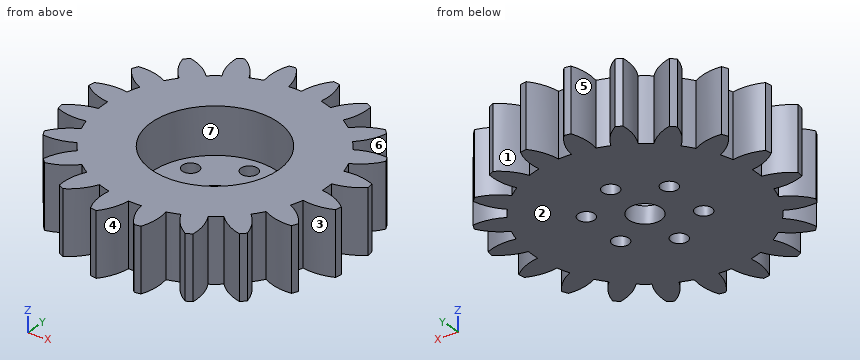
```python
from build123d import *

# Parameters (mm, degrees)
SKETCH1_R           = 3.25
BOSS_EXTRUDE1_DEPTH = 12.7
CUT_EXTRUDE1_REACH  = 43.167
SKETCH2_R           = 1.651
SKETCH3_R           = 12.7
CUT_EXTRUDE2_DEPTH  = 9.271


with BuildPart() as part:
    # Sketch1 → Boss-Extrude1 (new body)
    with BuildSketch(Plane.XY):
        with BuildLine():
            ThreePointArc((-27.689807384, 3.730705969), (-25.124393342, 2.086949602), (-22.186968024, 1.277742146))
            ThreePointArc((-22.186968024, 1.277742146), (-22.22373, 0), (-22.186968024, -1.277742146))
            ThreePointArc((-22.186968024, -1.277742146), (-25.124393342, -2.086949602), (-27.689807384, -3.730705969))
            ThreePointArc((-27.689807384, -3.730705969), (-27.596012236, -4.370778953), (-27.487423293, -5.00850883))
            ThreePointArc((-27.487423293, -5.00850883), (-24.539620899, -5.779057498), (-21.495904554, -5.640945179))
            ThreePointArc((-21.495904554, -5.640945179), (-21.136023233, -6.867510248), (-20.706216479, -8.071355168))
            ThreePointArc((-20.706216479, -8.071355168), (-23.249815112, -9.748671534), (-25.181720202, -12.104733275))
            ThreePointArc((-25.181720202, -12.104733275), (-24.894722286, -12.684494563), (-24.594378694, -13.257455889))
            ThreePointArc((-24.594378694, -13.257455889), (-21.552739385, -13.079370185), (-18.700672175, -12.007457487))
            ThreePointArc((-18.700672175, -12.007457487), (-17.979375248, -13.062780745), (-17.198596196, -14.074887709))
            ThreePointArc((-17.198596196, -14.074887709), (-19.099382988, -16.456125574), (-20.208670796, -19.293864949))
            ThreePointArc((-20.208670796, -19.293864949), (-19.756563466, -19.756563466), (-19.293864949, -20.208670796))
            ThreePointArc((-19.293864949, -20.208670796), (-16.456125574, -19.099382988), (-14.074887709, -17.198596196))
            ThreePointArc((-14.074887709, -17.198596196), (-13.062780745, -17.979375248), (-12.007457487, -18.700672175))
            ThreePointArc((-12.007457487, -18.700672175), (-13.079370185, -21.552739385), (-13.257455889, -24.594378694))
            ThreePointArc((-13.257455889, -24.594378694), (-12.684494563, -24.894722286), (-12.104733275, -25.181720202))
            ThreePointArc((-12.104733275, -25.181720202), (-9.748671534, -23.249815112), (-8.071355168, -20.706216479))
            ThreePointArc((-8.071355168, -20.706216479), (-6.867510248, -21.136023233), (-5.640945179, -21.495904554))
            ThreePointArc((-5.640945179, -21.495904554), (-5.779057498, -24.539620899), (-5.00850883, -27.487423293))
            ThreePointArc((-5.00850883, -27.487423293), (-4.370778953, -27.596012236), (-3.730705969, -27.689807384))
            ThreePointArc((-3.730705969, -27.689807384), (-2.086949602, -25.124393342), (-1.277742146, -22.186968024))
            ThreePointArc((-1.277742146, -22.186968024), (0, -22.22373), (1.277742146, -22.186968024))
            ThreePointArc((1.277742146, -22.186968024), (2.086949602, -25.124393342), (3.730705969, -27.689807384))
            ThreePointArc((3.730705969, -27.689807384), (4.370778953, -27.596012236), (5.00850883, -27.487423293))
            ThreePointArc((5.00850883, -27.487423293), (5.779057498, -24.539620899), (5.640945179, -21.495904554))
            ThreePointArc((5.640945179, -21.495904554), (6.867510248, -21.136023233), (8.071355168, -20.706216479))
            ThreePointArc((8.071355168, -20.706216479), (9.748671534, -23.249815112), (12.104733275, -25.181720202))
            ThreePointArc((12.104733275, -25.181720202), (12.684494563, -24.894722286), (13.257455889, -24.594378694))
            ThreePointArc((13.257455889, -24.594378694), (13.079370185, -21.552739385), (12.007457487, -18.700672175))
            ThreePointArc((12.007457487, -18.700672175), (13.062780745, -17.979375248), (14.074887709, -17.198596196))
            ThreePointArc((14.074887709, -17.198596196), (16.456125574, -19.099382988), (19.293864949, -20.208670796))
            ThreePointArc((19.293864949, -20.208670796), (19.756563466, -19.756563466), (20.208670796, -19.293864949))
            ThreePointArc((20.208670796, -19.293864949), (19.099382988, -16.456125574), (17.198596196, -14.074887709))
            ThreePointArc((17.198596196, -14.074887709), (17.979375248, -13.062780745), (18.700672175, -12.007457487))
            ThreePointArc((18.700672175, -12.007457487), (21.552739385, -13.079370185), (24.594378694, -13.257455889))
            ThreePointArc((24.594378694, -13.257455889), (24.894722286, -12.684494563), (25.181720202, -12.104733275))
            ThreePointArc((25.181720202, -12.104733275), (23.249815112, -9.748671534), (20.706216479, -8.071355168))
            ThreePointArc((20.706216479, -8.071355168), (21.136023233, -6.867510248), (21.495904554, -5.640945179))
            ThreePointArc((21.495904554, -5.640945179), (24.539620899, -5.779057498), (27.487423293, -5.00850883))
            ThreePointArc((27.487423293, -5.00850883), (27.596012236, -4.370778953), (27.689807384, -3.730705969))
            ThreePointArc((27.689807384, -3.730705969), (25.124393342, -2.086949602), (22.186968024, -1.277742146))
            ThreePointArc((22.186968024, -1.277742146), (22.22373, 0), (22.186968024, 1.277742146))
            ThreePointArc((22.186968024, 1.277742146), (25.124393342, 2.086949602), (27.689807384, 3.730705969))
            ThreePointArc((27.689807384, 3.730705969), (27.596012236, 4.370778953), (27.487423293, 5.00850883))
            ThreePointArc((27.487423293, 5.00850883), (24.539620899, 5.779057498), (21.495904554, 5.640945179))
            ThreePointArc((21.495904554, 5.640945179), (21.136023233, 6.867510248), (20.706216479, 8.071355168))
            ThreePointArc((20.706216479, 8.071355168), (23.249815112, 9.748671534), (25.181720202, 12.104733275))
            ThreePointArc((25.181720202, 12.104733275), (24.894722286, 12.684494563), (24.594378694, 13.257455889))
            ThreePointArc((24.594378694, 13.257455889), (21.552739385, 13.079370185), (18.700672175, 12.007457487))
            ThreePointArc((18.700672175, 12.007457487), (17.979375248, 13.062780745), (17.198596196, 14.074887709))
            ThreePointArc((17.198596196, 14.074887709), (19.099382988, 16.456125574), (20.208670796, 19.293864949))
            ThreePointArc((20.208670796, 19.293864949), (19.756563466, 19.756563466), (19.293864949, 20.208670796))
            ThreePointArc((19.293864949, 20.208670796), (16.456125574, 19.099382988), (14.074887709, 17.198596196))
            ThreePointArc((14.074887709, 17.198596196), (13.062780745, 17.979375248), (12.007457487, 18.700672175))
            ThreePointArc((12.007457487, 18.700672175), (13.079370185, 21.552739385), (13.257455889, 24.594378694))
            ThreePointArc((13.257455889, 24.594378694), (12.684494563, 24.894722286), (12.104733275, 25.181720202))
            ThreePointArc((12.104733275, 25.181720202), (9.748671534, 23.249815112), (8.071355168, 20.706216479))
            ThreePointArc((8.071355168, 20.706216479), (6.867510248, 21.136023233), (5.640945179, 21.495904554))
            ThreePointArc((5.640945179, 21.495904554), (5.779057498, 24.539620899), (5.00850883, 27.487423293))
            ThreePointArc((5.00850883, 27.487423293), (4.370778953, 27.596012236), (3.730705969, 27.689807384))
            ThreePointArc((3.730705969, 27.689807384), (2.086949602, 25.124393342), (1.277742146, 22.186968024))
            ThreePointArc((1.277742146, 22.186968024), (0, 22.22373), (-1.277742146, 22.186968024))
            ThreePointArc((-1.277742146, 22.186968024), (-2.086949602, 25.124393342), (-3.730705969, 27.689807384))
            ThreePointArc((-3.730705969, 27.689807384), (-4.370778953, 27.596012236), (-5.00850883, 27.487423293))
            ThreePointArc((-5.00850883, 27.487423293), (-5.779057498, 24.539620899), (-5.640945179, 21.495904554))
            ThreePointArc((-5.640945179, 21.495904554), (-6.867510248, 21.136023233), (-8.071355168, 20.706216479))
            ThreePointArc((-8.071355168, 20.706216479), (-9.748671534, 23.249815112), (-12.104733275, 25.181720202))
            ThreePointArc((-12.104733275, 25.181720202), (-12.684494563, 24.894722286), (-13.257455889, 24.594378694))
            ThreePointArc((-13.257455889, 24.594378694), (-13.079370185, 21.552739385), (-12.007457487, 18.700672175))
            ThreePointArc((-12.007457487, 18.700672175), (-13.062780745, 17.979375248), (-14.074887709, 17.198596196))
            ThreePointArc((-14.074887709, 17.198596196), (-16.456125574, 19.099382988), (-19.293864949, 20.208670796))
            ThreePointArc((-19.293864949, 20.208670796), (-19.756563466, 19.756563466), (-20.208670796, 19.293864949))
            ThreePointArc((-20.208670796, 19.293864949), (-19.099382988, 16.456125574), (-17.198596196, 14.074887709))
            ThreePointArc((-17.198596196, 14.074887709), (-17.979375248, 13.062780745), (-18.700672175, 12.007457487))
            ThreePointArc((-18.700672175, 12.007457487), (-21.552739385, 13.079370185), (-24.594378694, 13.257455889))
            ThreePointArc((-24.594378694, 13.257455889), (-24.894722286, 12.684494563), (-25.181720202, 12.104733275))
            ThreePointArc((-25.181720202, 12.104733275), (-23.249815112, 9.748671534), (-20.706216479, 8.071355168))
            ThreePointArc((-20.706216479, 8.071355168), (-21.136023233, 6.867510248), (-21.495904554, 5.640945179))
            ThreePointArc((-21.495904554, 5.640945179), (-24.539620899, 5.779057498), (-27.487423293, 5.00850883))
            ThreePointArc((-27.487423293, 5.00850883), (-27.596012236, 4.370778953), (-27.689807384, 3.730705969))
        make_face()
        Circle(SKETCH1_R, mode=Mode.SUBTRACT)
    extrude(amount=BOSS_EXTRUDE1_DEPTH)

    # Sketch2 → Cut-Extrude1 (cut, up to next)
    with BuildSketch(Plane.XY.offset(12.7), mode=Mode.PRIVATE) as cut_extrude1_sk1:
        with Locations((0, 9.5)):
            Circle(SKETCH2_R)
    cut_extrude1_tool1 = extrude(cut_extrude1_sk1.sketch, amount=-CUT_EXTRUDE1_REACH, mode=Mode.PRIVATE) & part.part
    # Sketch2 → Cut-Extrude1 (cut, up to next)
    with BuildSketch(Plane.XY.offset(12.7), mode=Mode.PRIVATE) as cut_extrude1_sk2:
        with Locations((8.227241336, 4.75)):
            Circle(SKETCH2_R)
    cut_extrude1_tool2 = extrude(cut_extrude1_sk2.sketch, amount=-CUT_EXTRUDE1_REACH, mode=Mode.PRIVATE) & part.part
    # Sketch2 → Cut-Extrude1 (cut, up to next)
    with BuildSketch(Plane.XY.offset(12.7), mode=Mode.PRIVATE) as cut_extrude1_sk3:
        with Locations((8.227241336, -4.75)):
            Circle(SKETCH2_R)
    cut_extrude1_tool3 = extrude(cut_extrude1_sk3.sketch, amount=-CUT_EXTRUDE1_REACH, mode=Mode.PRIVATE) & part.part
    # Sketch2 → Cut-Extrude1 (cut, up to next)
    with BuildSketch(Plane.XY.offset(12.7), mode=Mode.PRIVATE) as cut_extrude1_sk4:
        with Locations((0, -9.5)):
            Circle(SKETCH2_R)
    cut_extrude1_tool4 = extrude(cut_extrude1_sk4.sketch, amount=-CUT_EXTRUDE1_REACH, mode=Mode.PRIVATE) & part.part
    # Sketch2 → Cut-Extrude1 (cut, up to next)
    with BuildSketch(Plane.XY.offset(12.7), mode=Mode.PRIVATE) as cut_extrude1_sk5:
        with Locations((-8.227241336, -4.75)):
            Circle(SKETCH2_R)
    cut_extrude1_tool5 = extrude(cut_extrude1_sk5.sketch, amount=-CUT_EXTRUDE1_REACH, mode=Mode.PRIVATE) & part.part
    # Sketch2 → Cut-Extrude1 (cut, up to next)
    with BuildSketch(Plane.XY.offset(12.7), mode=Mode.PRIVATE) as cut_extrude1_sk6:
        with Locations((-8.227241336, 4.75)):
            Circle(SKETCH2_R)
    cut_extrude1_tool6 = extrude(cut_extrude1_sk6.sketch, amount=-CUT_EXTRUDE1_REACH, mode=Mode.PRIVATE) & part.part
    add(cut_extrude1_tool1.solids().sort_by_distance((0, 9.5, 12.7))[0], mode=Mode.SUBTRACT)
    add(cut_extrude1_tool2.solids().sort_by_distance((8.227241, 4.75, 12.7))[0], mode=Mode.SUBTRACT)
    add(cut_extrude1_tool3.solids().sort_by_distance((8.227241, -4.75, 12.7))[0], mode=Mode.SUBTRACT)
    add(cut_extrude1_tool4.solids().sort_by_distance((0, -9.5, 12.7))[0], mode=Mode.SUBTRACT)
    add(cut_extrude1_tool5.solids().sort_by_distance((-8.227241, -4.75, 12.7))[0], mode=Mode.SUBTRACT)
    add(cut_extrude1_tool6.solids().sort_by_distance((-8.227241, 4.75, 12.7))[0], mode=Mode.SUBTRACT)

    # Sketch3 → Cut-Extrude2 (cut)
    with BuildSketch(Plane.XY.offset(12.7)):
        Circle(SKETCH3_R)
    extrude(amount=-CUT_EXTRUDE2_DEPTH, mode=Mode.SUBTRACT)


solid = part.part
```
Check sheet for the modelled part. Datum: model origin and axes. Units: mm. Face numbers are marked on the shaded views. A direction names the side the tool comes from. Round coordinates to 2 decimals unless told otherwise and drop trailing zeros. Loops run counter-clockwise (first coordinate to the right, second up) from the corner with the lowest first, then second, coordinate; pieces in that order, holes last. Notation, with made-up numbers: (-34, -30) - (3, -30) arc R12 cw to (3, -21) - close; hole circle Ø1 at (-34, 10.5). An arc over 180 degrees is marked (long way). Answer as a JSON object with one key per item and string values. Group by question number.
Q1. Sectioned sample at A-A, the plane y = 0. Enter the section's corners in (x, z), plus the area to 3 significant figures.
Q2. Mould release check, pull along Y, two halves, no side actions. Record for the marked faces 1, 2, 3 and 4: released by +Y, released by -Y, zero draft, split by the parting line, or undercut.
Q3. Gauge pin test, flat ends, axial feed: P1, Ø4.5, axis at x = 0, y = 9.5, coming from the +Z side; P2, Ø5, axis at x = 21, z = 2.5, coming from the -Y side; P3, Ø6, axis at y = -7, z = 11, coming from the -X side; P4, Ø3, axis at x = 8.23, y = -4.75, coming from the +Z side. Record the tip position at first contact, or that the pin passes through.
Q4. Sectioned sample at B-B, the plane x = 0. Enter the section's corners in (y, z), plus the area to 3 significant figures.
Q5. Sectioned sample at C-C, the plane y = 9.5. Enter the section's corners in (x, z), plus the area to 3 significant figures.
Q6. Set-up check for the marked faces 5, 6 and 7: record each of +Z, -Z, +X, -X, +Y, -Y from which the full face is reachable in a straight line by a thin tool's end or side.
Q7. Scan lines: line 1 along Y through (x, z) = (-9.5, 3); line 2 along X through (y, z) = (-23, 0.5); line 3 along Y through (x, z) = (-17.5, 1.25). Record each from-to range of solid material in increasing order. Write a range as [from, to].
Solution:
{
 "1": {"outline": "(-22.22, 0) - (-3.25, 0) - (-3.25, 3.43) - (-12.7, 3.43) - (-12.7, 12.7) - (-22.22, 12.7) - close; (3.25, 0) - (22.22, 0) - (22.22, 12.7) - (12.7, 12.7) - (12.7, 3.43) - (3.25, 3.43) - close", "area": "307 mm²"},
 "2": {"face 1": "released by +Y", "face 2": "zero draft", "face 3": "undercut", "face 4": "released by -Y"},
 "3": {"P1": "stops at z = 3.43", "P2": "stops at y = -20.21", "P3": "stops at x = -27.65", "P4": "passes through"},
 "4": {"outline": "(-22.22, 0) - (-11.15, 0) - (-11.15, 3.43) - (-12.7, 3.43) - (-12.7, 12.7) - (-22.22, 12.7) - close; (-7.85, 0) - (-3.25, 0) - (-3.25, 3.43) - (-7.85, 3.43) - close; (3.25, 0) - (7.85, 0) - (7.85, 3.43) - (3.25, 3.43) - close; (11.15, 0) - (22.22, 0) - (22.22, 12.7) - (12.7, 12.7) - (12.7, 3.43) - (11.15, 3.43) - close", "area": "284 mm²"},
 "5": {"outline": "(-22.96, 0) - (-1.65, 0) - (-1.65, 3.43) - (-8.43, 3.43) - (-8.43, 12.7) - (-22.96, 12.7) - close; (1.65, 0) - (22.96, 0) - (22.96, 12.7) - (8.43, 12.7) - (8.43, 3.43) - (1.65, 3.43) - close", "area": "416 mm²"},
 "6": {"face 5": "+Z, -Z", "face 6": "+Z, -Z, +X", "face 7": "+Z"},
 "7": {"line 1": "y = [-22.96, -5.8], [-3.7, 3.7], [5.8, 22.96]", "line 2": "x = [-13.28, -9.53], [-5.82, -1.41], [1.41, 5.82], [9.53, 13.28]", "line 3": "y = [-19.62, -14.37], [-13.7, 13.7], [14.37, 19.62]"}
}
